Geometry check sheet. Reference: the model listing, model coordinates, mm. Face numbers are marked on the shaded views. A direction names the side the tool comes from. Give positions to 0.01 mm unless a question says otherwise; leave off trailing zeros. Order: outer loops, then holes, each group sorted by start corner. A loop starts at its lowest first (then second) coordinate and runs counter-clockwise, first axis right, second up.
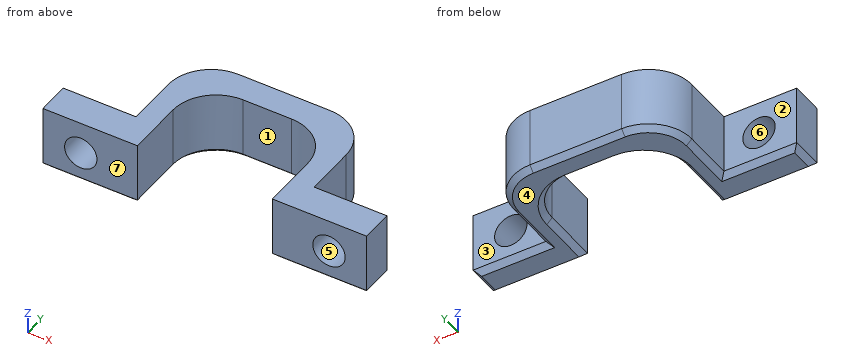
```python
from build123d import *

# Parameters (mm, degrees)
PAD_DEPTH    = 6
SKETCH001_R  = 1.5
POCKET_DEPTH = 5
FILLET_R     = 4
CHAMFER_SIZE = 0.5


with BuildPart() as part:
    # Sketch → Pad (new body)
    with BuildSketch(Plane.XY):
        Polygon((-15, 0), (-6.25, 0), (-6.25, 9.25), (6.25, 9.25), (6.25, 0), (15, 0), (15, 3), (8.25, 3), (8.25, 11.75), (-8.25, 11.75), (-8.25, 3), (-15, 3), align=None)
    extrude(amount=PAD_DEPTH)

    # Sketch001 → Pocket (cut)
    with BuildSketch(Plane.XZ):
        with Locations((-11.5, 3)):
            Circle(SKETCH001_R)
        with Locations((11.5, 3)):
            Circle(SKETCH001_R)
    extrude(amount=-POCKET_DEPTH, mode=Mode.SUBTRACT)

    # Fillet
    fillet_edges = [part.edges().sort_by_distance(p)[0] for p in [
        (6.25, 9.25, 3),
        (-6.25, 9.25, 3),
        (-8.25, 11.75, 3),
        (8.25, 11.75, 3),
    ]]
    fillet(fillet_edges, radius=FILLET_R)

    # Chamfer
    chamfer_edges = [part.edges().sort_by_distance(p)[0] for p in [
        (-6.25, 2.625, 0),
        (-5.078427, 8.078427, 0),
        (-10.625, 0, 0),
        (0, 9.25, 0),
        (-15, 1.5, 0),
        (5.078427, 8.078427, 0),
        (-11.625, 3, 0),
        (6.25, 2.625, 0),
        (-8.25, 5.375, 0),
        (10.625, 0, 0),
        (-7.078427, 10.578427, 0),
        (15, 1.5, 0),
        (0, 11.75, 0),
        (11.625, 3, 0),
        (7.078427, 10.578427, 0),
        (8.25, 5.375, 0),
    ]]
    chamfer(chamfer_edges, length=CHAMFER_SIZE)


solid = part.part
```
Q1. Access from +Z, -Z, +X, -X, +Y, -Y to the whole of each face (thin tool, end or side, straight path). Record for the marked faces 1, 2 and 3.
Q2. Cross-section at D-D, the plane z = 5.6. Record the boundary of the cut face in (x, y).
Q3. Gauge pin test, flat ends, axial feed: P1, Ø2.5, axis at y = 5, z = 4.5, coming from the +X side; P2, Ø1.6, axis at x = -12.5, z = 4.5, coming from the +Y side; P3, Ø2, axis at x = 5.5, z = 1.5, coming from the +Y side. Record the tip position at first contact, or that the pin passes through.
Q4. Cross-section at A-A, the plane y = 4.75. Record the boundary of the cut face in (x, z), and give its area (3 significant figures).
Q5. Thickness scan on L1, parallel to X at y = 0.75, z = 5.1; L2, parallel to Z at x = 11.5, y = 1.75; L3, parallel to X at y = 1.5, z = 2.55. Record the ranges inside material, lowest first.
Q6. Cross-section at C-C, the plane x = 11.5. Record the boundary of the cut face in (y, z), and give its area (3 significant figures).
Q7. Release check for a two-part mould opening along Z. For the marked faces 4, 5, 6 and 7 record: pulls with the +Z half, pulls with the -Z half, needs draft (parallel to the pull), parting line crosses it, or undercut.
Q8. Cross-section at B-B, the plane z = 4.2. Record the boundary of the cut face in (x, y), and give its area (3 significant figures).
Answers follow:
1. face 1: +Z, -Z, -Y
1. face 2: +Z, -Z, -X, +Y
1. face 3: +Z, -Z, +X, +Y
2. outline: (-15, 0) - (-6.25, 0) - (-6.25, 5.25) arc R4 cw to (-2.25, 9.25) - (2.25, 9.25) arc R4 cw to (6.25, 5.25) - (6.25, 0) - (15, 0) - (15, 3) - (8.25, 3) - (8.25, 7.75) arc R4 ccw to (4.25, 11.75) - (-4.25, 11.75) arc R4 ccw to (-8.25, 7.75) - (-8.25, 3) - (-15, 3) - close
3. P1: stops at x = 8.25
3. P2: stops at y = 3
3. P3: stops at y = 11.74
4. outline: (-8.25, 0.5) - (-7.75, 0) - (-6.75, 0) - (-6.25, 0.5) - (-6.25, 6) - (-8.25, 6) - close; (6.25, 0.5) - (6.75, 0) - (7.75, 0) - (8.25, 0.5) - (8.25, 6) - (6.25, 6) - close
4. area: 23.5 mm2
5. L1: x = -15 to -6.25, 6.25 to 15
5. L2: z = 0 to 1.5, 4.5 to 6
5. L3: x = -15 to -12.93, -10.07 to -6.25, 6.25 to 10.07, 12.93 to 15
6. outline: (0, 0.5) - (0.5, 0) - (2.5, 0) - (3, 0.5) - (3, 1.5) - (0, 1.5) - close; (0, 4.5) - (3, 4.5) - (3, 6) - (0, 6) - close
6. area: 8.75 mm2
7. face 4: pulls with the -Z half
7. face 5: undercut
7. face 6: undercut
7. face 7: needs draft
8. outline: (-15, 0) - (-12.4, 0) - (-12.4, 3) - (-15, 3) - close; (-10.6, 0) - (-6.25, 0) - (-6.25, 5.25) arc R4 cw to (-2.25, 9.25) - (2.25, 9.25) arc R4 cw to (6.25, 5.25) - (6.25, 0) - (10.6, 0) - (10.6, 3) - (8.25, 3) - (8.25, 7.75) arc R4 ccw to (4.25, 11.75) - (-4.25, 11.75) arc R4 ccw to (-8.25, 7.75) - (-8.25, 3) - (-10.6, 3) - close; (12.4, 0) - (15, 0) - (15, 3) - (12.4, 3) - close
8. area: 108 mm2
